CAD build for the part. Positions are in the model's coordinates, mm. Face numbers are marked on the shaded views. A direction names the side the tool comes from. Give positions to 0.01 mm unless a question says otherwise; leave off trailing zeros. Write each loop counter-clockwise with the first axis right and the second up, starting at its lowest first coordinate (ties: lowest second). Pieces come first, ordered by that corner, then holes. Notation, with made-up numbers: (67, 10.25) - (100, 10.25) arc R21 cw to (100, 43.25) - close; hole circle Ø7 at (-33.75, 13). An arc over 180 degrees is marked (long way). Answer as a JSON object with one key per item and string values.
Autodesk Inventor part; units mm, degrees
ref_plane "YZ Plane" through (0, 0, 0) normal (1, 0, 0) x (0, 1, 0)
ref_plane "XZ Plane" through (0, 0, 0) normal (0, 1, 0) x (-1, 0, 0)
ref_plane "XY Plane" through (0, 0, 0) normal (0, 0, 1) x (1, 0, 0)
sketch "Szkic1" plane through (0, 0, 0) normal (0, 1, 0) x (-1, 0, 0)
  circle A0 centre (0, 0) radius 2.5
  circle A1 centre (0, 0) radius 8
  circle A2 centre (0, 0) radius 3.5
  circle A3 centre (0, 0) radius 3.5
  circle A4 centre (0, 0) radius 6.75
  circle A5 centre (0, 0) radius 5
  circle A6 centre (0, 0) radius 3.75
  dimension "d0" = 5
  dimension "d1" = 16
  dimension "d2" = 7
  dimension "d3" = 7
  dimension "d4" = 13.5
  dimension "d13" = 10
  dimension "d16" = 7.5
extrude "Wyciągnięcie proste7" add sketch "Szkic1" along normal mid plane 4.5 contours A2
extrude "Wyciągnięcie proste8" add sketch "Szkic1" along normal mid plane 4.75 contours A5
extrude "Wyciągnięcie proste9" add sketch "Szkic1" along normal mid plane 1.5 contours A0 | A2 | A6
extrude "Wyciągnięcie proste10" add sketch "Szkic1" along normal mid plane 5 contours A1
extrude "Wyciągnięcie proste11" add sketch "Szkic1" along normal mid plane 4.75 contours A4
sketch "Szkic2" plane through (0, 0.75, 0) normal (0, 1, 0) x (1, 0, 0)
  point P0 (0, 0)
  point P1 (0.0085, 0.051)
hole "Otwór3" at (0, 0.75, 0) direction (0, -1, 0) diameter 5 end through all
chamfer "Faza3" distance 0.125 angle 45 1 edges at (2.5, 2.25, 0)
properties part number "lozysko"
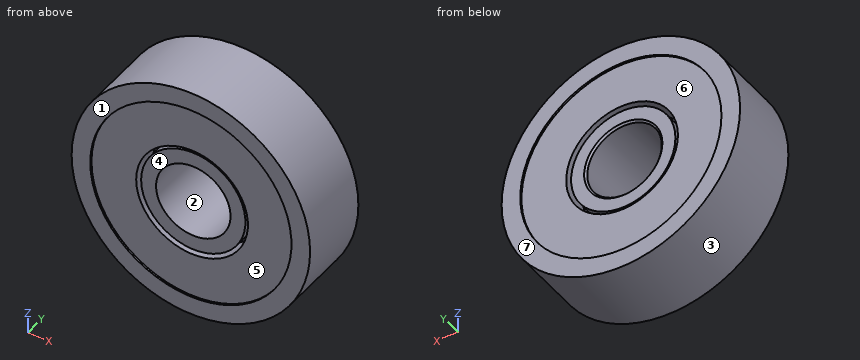
Item 1: Cut at B-B (x = -4.75). Give the cut face in (y, z) (3 decimals), and give its area (3 significant figures).
Entries:
{"outline": "(-2.5, -6.437) - (2.5, -6.437) - (2.5, -4.796) - (2.375, -4.796) - (2.375, 4.796) - (2.5, 4.796) - (2.5, 6.437) - (-2.5, 6.437) - (-2.5, 4.796) - (-2.375, 4.796) - (-2.375, -4.796) - (-2.5, -4.796) - close", "area": "62.0 mm2"}
Item 2: Flat gauge pins, fed straight in: P1, Ø1.5, axis at x = 5, y = -1, coming from the -Z side; P2, Ø6.5, axis at x = 0, z = 0, coming from the +Y side; P3, Ø3.5, axis at x = 1, z = -1, coming from the -Y side. Where does each tip first touch, or does it go through?
Entries:
{"P1": "z = -6.78", "P2": "y = 2.25", "P3": "y = -2.25"}
Item 3: Cut at A-A (y = -1.45). Give the cut face in (x, z).
Entries:
{"outline": "circle Ø16 at (0, 0); circle Ø7 at (0, 0); hole circle Ø7.5 at (0, 0); hole circle Ø5 at (0, 0)"}
Item 4: Cut at D-D (x = -7). Give the cut face in (y, z), and give its area (3 significant figures).
Entries:
{"outline": "(-2.5, -3.87) - (2.5, -3.87) - (2.5, 3.87) - (-2.5, 3.87) - close", "area": "38.7 mm2"}
Item 5: Cut at C-C (z = 5.75). Give the cut face in (x, y) (3 decimals).
Entries:
{"outline": "(-5.562, -2.5) - (-3.536, -2.5) - (-3.536, -2.375) - (3.536, -2.375) - (3.536, -2.5) - (5.562, -2.5) - (5.562, 2.5) - (3.536, 2.5) - (3.536, 2.375) - (-3.536, 2.375) - (-3.536, 2.5) - (-5.562, 2.5) - close"}
Item 6: Probe line 1 (Z direction, x = 0, y = -0.45); line 2 (Z direction, x = 0.75, y = 1.3); line 3 (Z direction, x = 0.25, y = -1.4). List the from-to ranges inside material, lowest first. Write a range as from..to.
Entries:
{"line 1": "-8..-2.5, 2.5..8", "line 2": "-7.96..-3.67, -3.42..-2.38, 2.38..3.42, 3.67..7.96", "line 3": "-8..-3.74, -3.49..-2.49, 2.49..3.49, 3.74..8"}
Item 7: Which spindle directions (+Z, -Z, +X, -X, +Y, -Y) get a long thin tool onto all of the face, cutting with end or side? Do the marked faces 5, 6 and 7. Say none if no direction does.
Entries:
{"face 5": "-Y", "face 6": "+Y", "face 7": "+Z, -Z, +X, -X, +Y"}
Item 8: Mould opens along X. For the marked faces 1, 2, 3 and 4 say: +X half, -X half, draft (parallel to the pull), parting line (faces both ways), or undercut.
Entries:
{"face 1": "draft", "face 2": "undercut", "face 3": "parting line", "face 4": "undercut"}
